from build123d import *

# Parameters (mm, degrees)
SKETCH014_R  = 1.75
PAD008_DEPTH = 0.1
SKETCH015_R  = 3
PAD009_DEPTH = 12.9
CHAMFER_SIZE = 1


with BuildPart() as part:
    # Sketch014 → Pad008 (new body)
    with BuildSketch(Plane.XZ):
        Circle(SKETCH014_R)
    extrude(amount=PAD008_DEPTH)

    # Sketch015 (on Face3 of Pad008) → Pad009 (join)
    with BuildSketch(Plane.XZ.offset(0.1)):
        Circle(SKETCH015_R)
    extrude(amount=PAD009_DEPTH)

    # Chamfer
    chamfer_edges = [part.edges().sort_by_distance(p)[0] for p in [
        (-3, -13, 0),
    ]]
    chamfer(chamfer_edges, length=CHAMFER_SIZE)


with BuildPart() as part_1:
    # Body002 placement: moved
    add(part.part.moved(Location((0, -9.5, 0))))


solid = part_1.part
Can you work these out from the model? Positions are in its coordinate system, mm. A direction names the side the tool comes from. Give positions to 0.01 mm unless a question says otherwise; leave off trailing zeros. Loops run counter-clockwise (first coordinate to the right, second up) from the corner with the lowest first, then second, coordinate; pieces in that order, holes last. Notation, with made-up numbers: M 7.25,63 L 39.25,63 A10 ccw 39.25,72 Z; hole C 71.5,-26.5 d10. An arc over 180 degrees is marked long. One line per item, written item: value.
1) I'm going to push flat-ended pins straight in: pin 1 (1.5 mm diameter, centred on y = -19.5, z = -1.5, fed in from -X); pin 2 (3 mm diameter, centred on y = -19, z = 2, fed in from +X). Where does each tip first touch, or does it pass through?
Geometry check:
pin 1: stops at x = -2.9
pin 2: stops at x = 2.96
2) On a 3-axis mill with a long thin cutter (end or side, diameter ignored), from which of +Z, -Z, +X, -X, +Y, -Y can I reach the whole of each face in a straight line? I mean faces 1 (the face through (0, -9.5, 0)), 2 (the face through (0, -9.6, -2)). Say none if no direction works.
Geometry check:
face 1: +Z, -Z, +X, -X, +Y
face 2: +Y
3) Imagine slicing it at C-C on y = -16.25. Write out the boundary of the cut face in (x, z).
Geometry check:
outline: C 0,0 d6
4) Imagine slicing it at A-A on z = 0. Write out the boundary of the cut face in (x, y).
Geometry check:
outline: M -3,-21.5 L -2,-22.5 L 2,-22.5 L 3,-21.5 L 3,-9.6 L 1.75,-9.6 L 1.75,-9.5 L -1.75,-9.5 L -1.75,-9.6 L -3,-9.6 Z
5) Please list where these lines run through material, in increasing order: line 1 (Z direction, x = -0.1, y = -17.5); line 2 (X direction, y = -19.25, z = -0.55); line 3 (Z direction, x = -2.1, y = -21).
Geometry check:
line 1: z = -3 to 3
line 2: x = -2.95 to 2.95
line 3: z = -2.14 to 2.14
6) Imagine slicing it at B-B on x = 0. Write out the boundary of the cut face in (y, z), and give its area (4 significant figures).
Geometry check:
outline: M -22.5,-2 L -21.5,-3 L -9.6,-3 L -9.6,-1.75 L -9.5,-1.75 L -9.5,1.75 L -9.6,1.75 L -9.6,3 L -21.5,3 L -22.5,2 Z
area: 76.75 mm²
